Geometry: final body of the model. Coordinates: model frame, mm. Give positions to 0.01 mm unless a question says otherwise; leave off trailing zeros. Order: outer loops, then holes, each group sorted by start corner. A loop starts at its lowest first (then second) coordinate and runs counter-clockwise, first axis right, second up. Notation, with made-up numbers: (81, -7) -> (85, -7) arc R31 cw to (85, 28) -> close; hole circle Ø8 at (-14, 63.5). An arc over 180 degrees is marked (long way). One line per question, with ' | ' between items.
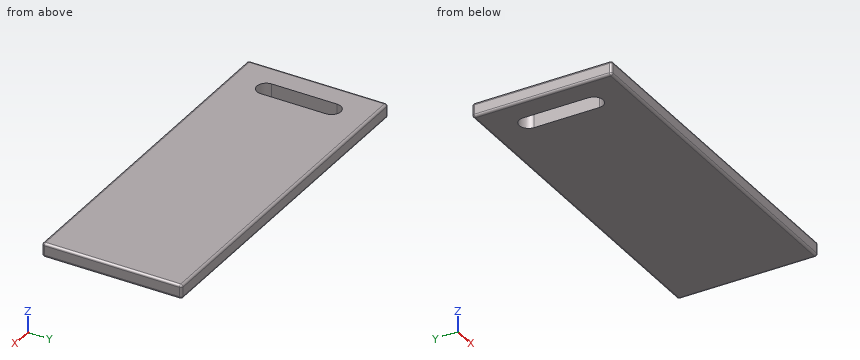
from build123d import *

# Parameters (mm, degrees)
F0_W     = 75
F0_H     = 30
F1_DEPTH = 3
F2_W     = 4
F2_H     = 7
F3_DEPTH = 25
F4_R     = 0.5


with BuildPart() as f1:
    # F0 (on Top) → F1 (new body)
    with BuildSketch(Plane.XY):
        with Locations((37.5, 15)):
            Rectangle(F0_W, F0_H)
    extrude(amount=F1_DEPTH)

    # F2 (on face) → F3 (cut)
    with BuildSketch(Plane.XY.offset(3)):
        with BuildLine():
            Line((5, 22), (5, 15))
            Line((5, 15), (9, 15))
            Line((9, 15), (9, 22))
            ThreePointArc((9, 22), (7, 24), (5, 22))
        make_face()
        with Locations((7, 11.5)):
            Rectangle(F2_W, F2_H)
        with BuildLine():
            Line((9, 8), (5, 8))
            ThreePointArc((5, 8), (7, 6), (9, 8))
        make_face()
    extrude(amount=-F3_DEPTH, mode=Mode.SUBTRACT)

    # F4
    f4_edges = [f1.edges().sort_by_distance(p)[0] for p in [
        (37.5, 30, 3),
        (0, 15, 3),
        (37.5, 0, 3),
        (75, 15, 3),
        (75, 15, 0),
        (37.5, 0, 0),
        (37.5, 30, 0),
        (0, 15, 0),
        (75, 0, 1.5),
        (75, 30, 1.5),
        (0, 30, 1.5),
        (0, 0, 1.5),
    ]]
    fillet(f4_edges, radius=F4_R)


solid = f1.part
1) Section C-C on y = 13.25. Return loops of the section in (x, z).
Check result:
outline: (0, 0.5) arc R0.5 ccw to (0.5, 0) -> (5, 0) -> (5, 3) -> (0.5, 3) arc R0.5 ccw to (0, 2.5) -> close; (9, 0) -> (74.5, 0) arc R0.5 ccw to (75, 0.5) -> (75, 2.5) arc R0.5 ccw to (74.5, 3) -> (9, 3) -> close
2) Section B-B on x = 7. Return loops of the section in (y, z), plus the area to 3 significant figures.
Check result:
outline: (0, 0.5) arc R0.5 ccw to (0.5, 0) -> (6, 0) -> (6, 3) -> (0.5, 3) arc R0.5 ccw to (0, 2.5) -> close; (24, 0) -> (29.5, 0) arc R0.5 ccw to (30, 0.5) -> (30, 2.5) arc R0.5 ccw to (29.5, 3) -> (24, 3) -> close | area: 35.8 mm^2
3) Material intervals for probe 1 along X at (y, z) = (15.75, 0.7); probe 2 along X at (y, z) = (25, 0.45); probe 3 along Y at (x, z) = (32.5, 2.55), sorted ascending. Write a range as from..to.
Check result:
probe 1: x = 0..5, 9..75 | probe 2: x = 0..75 | probe 3: y = 0..30
4) Section A-A on z = 1.95. Return loops of the section in (x, y).
Check result:
outline: (0, 0.5) arc R0.5 ccw to (0.5, 0) -> (74.5, 0) arc R0.5 ccw to (75, 0.5) -> (75, 29.5) arc R0.5 ccw to (74.5, 30) -> (0.5, 30) arc R0.5 ccw to (0, 29.5) -> close; hole (5, 8) arc R2 ccw to (9, 8) -> (9, 22) arc R2 ccw to (5, 22) -> close
